For this review, take the finished solid that the model builds, in its own axes (mm). A direction names the side the tool comes from. Round coordinates to 2 decimals unless told otherwise and drop trailing zeros. Write each loop counter-clockwise with the first axis right and the second up, starting at its lowest first coordinate (ties: lowest second). Pieces come first, ordered by that corner, then holes. Notation, with made-up numbers: M -4,76.5 L 23,76.5 A21 ccw 23,113.5 Z; hole C 49.5,23.5 d1. An arc over 180 degrees is marked long. Answer in a Markdown table with one row per item.
```python
from build123d import *

# Parameters (mm, degrees)
F0_W      = 25
F0_H      = 120
F1_DEPTH  = 10
F3_W      = 3
F3_H      = 114
F4_DEPTH  = 25.001
F5_W      = 9.2
F5_H      = 100
F6_DEPTH  = 7.2
F7_R      = 2.6
F8_DEPTH  = 105.001
F9_W      = 4
F9_H      = 100
F10_DEPTH = 3
F11_W     = 7.2
F11_H     = 60
F12_DEPTH = 17.101
F13_W     = 25
F13_H     = 85
F14_DEPTH = 3.5
F15_W     = 3
F15_H     = 85
F16_DEPTH = 3.5
F17_R     = 2


with BuildPart() as f1:
    # F0 (on Front) → F1 (new body)
    with BuildSketch(Plane.XZ):
        Rectangle(F0_W, F0_H)
    extrude(amount=F1_DEPTH)

    # F3 (on face) → F4 (cut, through all)
    with BuildSketch(Plane.YZ.offset(12.5)):
        with Locations((-5, -3)):
            Rectangle(F3_W, F3_H)
    extrude(amount=-F4_DEPTH, mode=Mode.SUBTRACT)

    # F5 (on face) → F6 (join)
    with BuildSketch(Plane(origin=(0, 0, 0), x_dir=(-1, 0, 0), z_dir=(0, 1, 0))):
        with Locations((0, -5)):
            Rectangle(F5_W, F5_H)
    extrude(amount=F6_DEPTH)

    # F7 (on face) → F8 (cut, through all)
    with BuildSketch(Plane.XY.offset(45)):
        with Locations((0, 2.785714576)):
            Circle(F7_R)
    extrude(amount=-F8_DEPTH, mode=Mode.SUBTRACT)

    # F9 (on face) → F10 (cut)
    with BuildSketch(Plane(origin=(0, 7.2, 0), x_dir=(-1, 0, 0), z_dir=(0, 1, 0))):
        with Locations((0, -5)):
            Rectangle(F9_W, F9_H)
    extrude(amount=-F10_DEPTH, mode=Mode.SUBTRACT)

    # F11 (on face) → F12 (cut, through all)
    with BuildSketch(Plane.YZ.offset(4.6)):
        with Locations((3.6, -5)):
            Rectangle(F11_W, F11_H)
    extrude(amount=-F12_DEPTH, mode=Mode.SUBTRACT)

    # F13 (on face) → F14 (cut, through all)
    with BuildSketch(Plane.XZ.offset(10)):
        with Locations((0, -17.5)):
            Rectangle(F13_W, F13_H)
    extrude(amount=-F14_DEPTH, mode=Mode.SUBTRACT)

    # F15 (on face) → F16 (cut, through all)
    with BuildSketch(Plane(origin=(0, 0, 0), x_dir=(-1, 0, 0), z_dir=(0, 1, 0))):
        with Locations((-11, -17.5)):
            Rectangle(F15_W, F15_H)
        with Locations((11, -17.5)):
            Rectangle(F15_W, F15_H)
    extrude(amount=-F16_DEPTH, mode=Mode.SUBTRACT)

    # F17
    f17_edges = [f1.edges().sort_by_distance(p)[0] for p in [
        (-12.5, -8.25, 25),
        (-12.5, -1.75, 25),
        (12.5, -1.75, 25),
        (12.5, -8.25, 25),
        (-12.5, -5, 60),
        (12.5, -5, 60),
        (-9.5, -1.75, -60),
        (9.5, -1.75, -60),
        (-4.6, 7.2, 35),
        (4.6, 7.2, 35),
        (-4.6, 0, 35),
        (4.6, 0, 35),
        (-4.6, 7.2, -45),
        (4.6, 7.2, -45),
        (-4.6, 0, -45),
        (4.6, 0, -45),
    ]]
    fillet(f17_edges, radius=F17_R)


solid = f1.part
```
Q1. Take a section at B-B (x = 0). State the section outline as (y, z) points, then the cut area to 3 significant figures.
Found:
| item | result |
|---|---|
| outline | M -10,25 L -6.5,25 L -6.5,54 L -3.5,54 L -3.5,-60 L 0,-60 L 0,-55 L 0.19,-55 L 0.19,-35 L 0,-35 L 0,25 L 0.19,25 L 0.19,45 L 0,45 L 0,60 L -10,60 Z |
| area | 568 mm² |
Q2. Machinability: for faces 1 (the face through (-4.6, 4, -45)), 2 (the face through (-3, 3, -35)), 3 (the face through (4.6, 4, -45)), 4 (the face through (-2, 6, -45)), 5 (the face through (0, -5, 54)), which of the approach directions +Z, -Z, +X, -X, +Y, -Y give a long, thin tool a straight path to every point of the face, cutting with its end or side? Answer none if there is none.
Found:
| item | result |
|---|---|
| face 1 | +Z, -Z, -X, +Y |
| face 2 | +X, -X, +Y |
| face 3 | +Z, -Z, +X, +Y |
| face 4 | +Z, -Z, +Y |
| face 5 | -Z, +X, -X |
Q3. Mouldability with a two-part tool opening along Y and no side actions: class faces 6 (the face through (-5.2, 0.57, 35.14)), 7 (the face through (-3, 3, 45)), 8 (the face through (0, -3.5, -4)) as +Y half, -Y half, draft (parallel to the pull), parting line (faces both ways), or undercut.
Found:
| item | result |
|---|---|
| face 6 | +Y half |
| face 7 | draft |
| face 8 | undercut |
Q4. Take a section at A-A (y = 3.25). State the section outline as (x, z) points, then the cut area to 3 significant figures.
Found:
| item | result |
|---|---|
| outline | M -4.6,-55 L -2.56,-55 L -2.56,-35 L -4.6,-35 Z; M -4.6,25 L -2.56,25 L -2.56,45 L -4.6,45 Z; M 2.56,-55 L 4.6,-55 L 4.6,-35 L 2.56,-35 Z; M 2.56,25 L 4.6,25 L 4.6,45 L 2.56,45 Z |
| area | 163 mm² |
Q5. Take a section at D-D (z = 21). State the section outline as (x, y) points.
Found:
| item | result |
|---|---|
| outline | M -9.5,-3.5 L 9.5,-3.5 L 9.5,0 L -9.5,0 Z |
Q6. Take a section at C-C (y = -1.25). State the section outline as (x, z) points.
Found:
| item | result |
|---|---|
| outline | M -12.5,27 A2 ccw -10.5,25 L -9.5,25 L -9.5,-58 A2 ccw -7.5,-60 L 7.5,-60 A2 ccw 9.5,-58 L 9.5,25 L 10.5,25 A2 ccw 12.5,27 L 12.5,58 A2 ccw 10.5,60 L -10.5,60 A2 ccw -12.5,58 Z |
Q7. Insertion check: P1, Ø8, axis at y = 0, z = -19.5, coming from the +X side; P2, Ø1, axis at y = 3, z = 37, coming from the -X side; P3, Ø6, axis at x = 1.5, y = 2, coming from the +Z side; P4, Ø1.8, axis at y = -1.5, z = -37, coming from the -X side. Each pin has a flat end and moves straight along its axis. Give the tip position at first contact, or say it passes through.
Found:
| item | result |
|---|---|
| P1 | x = 9.5 |
| P2 | x = -4.6 |
| P3 | z = 60 |
| P4 | x = -9.5 |
Q8. For probe 1 along Y at (x, z) = (2.25, 45.5); probe 2 along X at (y, z) = (4.5, 32); probe 3 along Y at (x, z) = (0, 31), list the stretches that pass through material, from the lowest coordinate up.
Found:
| item | result |
|---|---|
| probe 1 | -10 to -6.5, -3.5 to 0 |
| probe 2 | -4.6 to -2, 2 to 4.6 |
| probe 3 | -10 to -6.5, -3.5 to 0.19 |
